Geometry: final body of the model. Coordinates: model frame, mm. Face numbers are marked on the shaded views. A direction names the side the tool comes from. Give positions to 0.01 mm unless a question says otherwise; leave off trailing zeros. Write each loop counter-clockwise with the first axis right and the second up, starting at its lowest first coordinate (ties: lowest second). Pieces come first, ordered by that corner, then holes. Notation, with made-up numbers: M 28,-14 L 52,-14 A15 cw 52,-3 Z; hole C 36,25.5 d4. An arc over 180 degrees is marked long. Use one line per item in the form item = value. Start each with the question number.
Item 1: Section query A-A on y = 0. Return loops of the section in (x, z), then the cut area to 3 significant figures.
Item 2: Section query D-D on z = 9.75. Return loops of the section in (x, y), then the cut area to 3 significant figures.
Item 3: Section query C-C on z = 3. Return loops of the section in (x, y), then the cut area to 3 significant figures.
Item 4: Access query for the marked faces 5 and 6. Directions: +Z, -Z, +X, -X, +Y, -Y. A direction counts if a zero-diameter tool reaches every point of the face in a straight line with its end or side. Return the directions, or none.
Item 5: Material intervals for line 1 along X through (y, z) = (-0.25, 13); line 2 along Z through (x, y) = (-2.25, 4.5), sorted ascending. Write a range as from..to.
Item 6: Contact query for flat-ended pins moving along their axis: P1, Ø4, axis at y = 4, z = 3, coming from the -X side; P2, Ø3, axis at x = -3, z = 6, coming from the +Y side; P3, Ø1, axis at x = -5.5, z = 6.5, coming from the -Y side. Output: stop coordinate, or through.
Item 7: Pull-direction query (Z, two-part tool) for the marked faces 1, 2, 3 and 4; classes: released by +Z, released by -Z, zero draft, split by the parting line, or undercut.
Autodesk Fusion 360 part; units mm, degrees
sketch "Sketch1" plane through (0, 0, 0) normal (0, 0, 1) x (1, 0, 0)
  circle A0 centre (0, 0) radius 6.65
  circle A1 centre (0, 0) radius 9.65
  dimension "d1" = 13.3
  dimension "d2" = 3
extrude "Extrude1" add sketch "Sketch1" along normal blind 15
extrude "Extrude2" add sketch "Sketch1" along normal blind 5 contours A0
sketch "Sketch2" plane through (0, 0, 0) normal (0, 0, 1) x (1, 0, 0)
  circle A0 centre (0, 0) radius 9.65
  dimension "d7" = 19.3
extrude "Extrude3" add sketch "Sketch2" against normal blind 7
sketch "Sketch3" plane through (0, 0, -7) normal (0, 0, -1) x (1, 0, 0)
  circle A0 centre (0, 0) radius 9.65
  circle A1 centre (0, 0) radius 5
  dimension "d10" = 10
chamfer "Chamfer1" distance 1 angle 45 1 edges at (-8.997, 3.4896, -7)
sketch "Sketch4" plane through (0, 0, 0) normal (0, 1, 0) x (1, 0, 0)
  line L0 (9.65, 6) -> (-9.65, 6)
  line L1 (9.65, 6) -> (9.65, 0)
  line L2 (9.65, 0) -> (6.65, 3)
  line L3 (6.65, 3) -> (9.65, 6)
  line L4 (0, 0) -> (9.65, 0)
  dimension "d18" = 45
revolve "Revolve1" cut sketch "Sketch4" angle 360 about axis through (0, 0, 1.75) along (0, 0, 1)
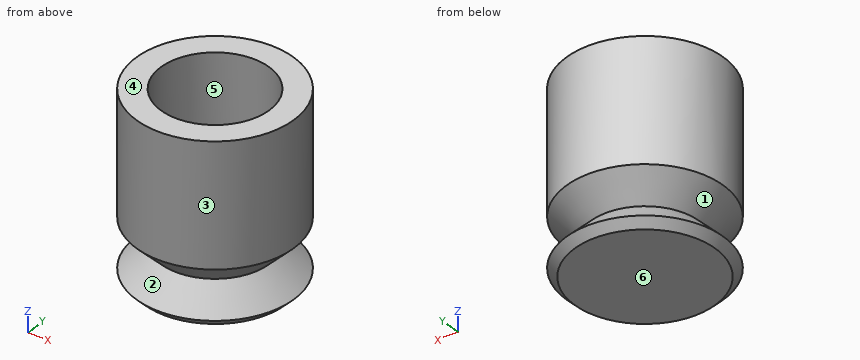
Answer sheet:
q1.outline = M -9.65,-6 L -8.65,-7 L 8.65,-7 L 9.65,-6 L 6.65,-3 L 9.65,0 L 9.65,15 L 6.65,15 L 6.65,5 L -6.65,5 L -6.65,15 L -9.65,15 L -9.65,0 L -6.65,-3 Z
q1.area = 273 mm2
q2.outline = C 0,0 d19.3; hole C 0,0 d13.3
q2.area = 154 mm2
q3.outline = C 0,0 d19.3
q3.area = 293 mm2
q4.face_5 = +Z
q4.face_6 = -Z, +X, -X, +Y, -Y
q5.line_1 = -9.65..-6.65, 6.65..9.65
q5.line_2 = -7..5
q6.P1 = -9.44
q6.P2 = 9.53
q6.P3 = -8.25
q7.face_1 = undercut
q7.face_2 = undercut
q7.face_3 = zero draft
q7.face_4 = released by +Z
